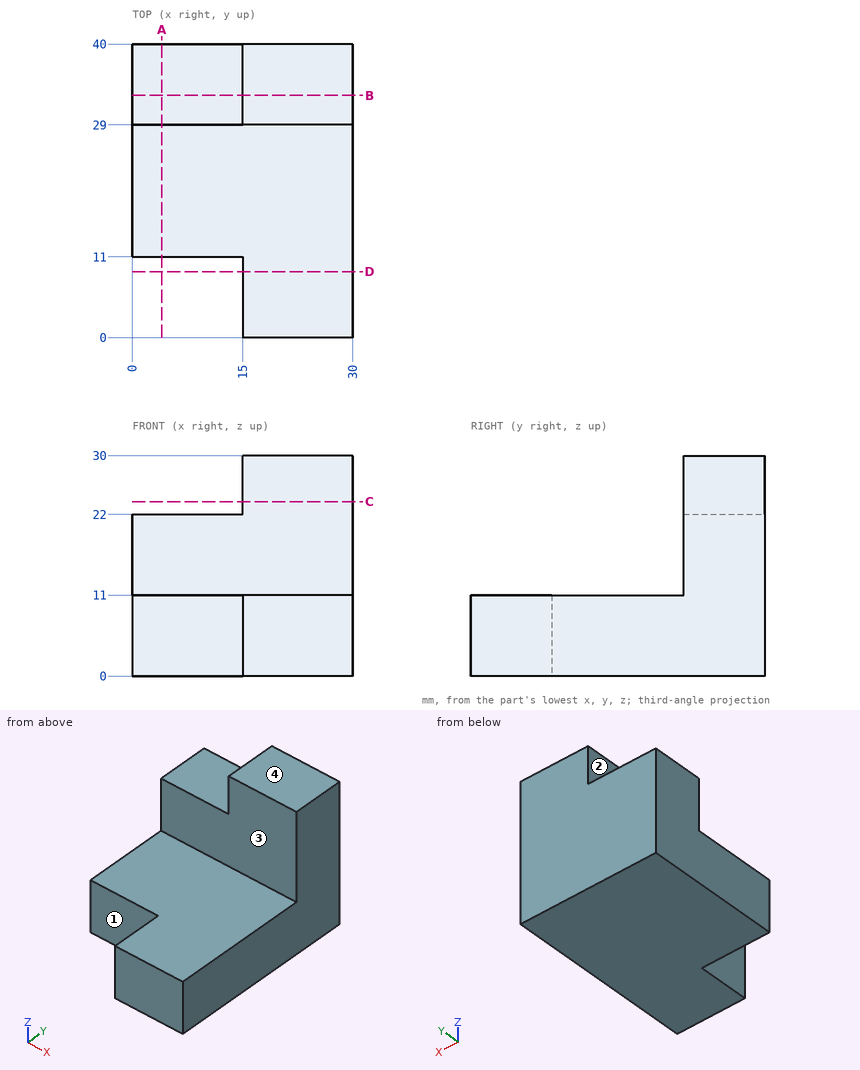
The drawing under review shows one solid part. Ordinate dimensions are in mm from its lowest x, y, z. A direction names the side the tool comes from. Round coordinates to 2 decimals unless told otherwise and drop trailing zeros. Loops run counter-clockwise (first coordinate to the right, second up) from the corner with the lowest first, then second, coordinate; pieces in that order, holes last. Notation, with made-up numbers: (50.5, 33) - (109.5, 33) arc R30 ccw to (109.5, 66) - close; hole circle Ø4 at (52, -27.75). An arc over 180 degrees is marked (long way). Put each result on its own line as item: value. Start each with the question number.
1. Consider section A-A on x = 4. State the section outline as (y, z) points.
2. For probe 1 along Z at (x, y) = (15, 18); probe 2 along Y at (x, z) = (15, 19); probe 3 along Z at (x, y) = (8, 30.5), list the stretches that pass through material, from the lowest coordinate up. Write a range as [from, to].
3. Consider section B-B on y = 33. State the section outline as (x, z) points, plus the area to 3 significant figures.
4. Consider section C-C on z = 23.75. State the section outline as (x, y) points, plus the area to 3 significant figures.
5. For the marked faces 1, 2, 3 and 4, list the 3-axis set-ups (+Z, -Z, +X, -X, +Y, -Y) from which the entire face can be reached by the end or side of a thin tool; tool diameter is ignored.
6. Consider section D-D on y = 9. State the section outline as (x, z) points, plus the area to 3 significant figures.
7. Insertion check: P1, Ø12, axis at x = 6, z = 7.5, coming from the -Y side; P2, Ø12, axis at x = 8, y = 34.5, coming from the +Z side; P3, Ø2, axis at x = 4.5, y = 16.5, coming from the +Z side. Each pin has a flat end and moves straight along its axis. Give the tip position at first contact, or say it passes through.
Result sheet:
1. outline: (11, 0) - (40, 0) - (40, 22) - (29, 22) - (29, 11) - (11, 11) - close
2. probe 1: [0, 11]
2. probe 2: [29, 40]
2. probe 3: [0, 22]
3. outline: (0, 0) - (30, 0) - (30, 30) - (15, 30) - (15, 22) - (0, 22) - close
3. area: 780 mm^2
4. outline: (15, 29) - (30, 29) - (30, 40) - (15, 40) - close
4. area: 165 mm^2
5. face 1: +Z, -Z, -X, -Y
5. face 2: +Z, -X, +Y, -Y
5. face 3: +Z, +X, -X, -Y
5. face 4: +Z, +X, -X, +Y, -Y
6. outline: (15, 0) - (30, 0) - (30, 11) - (15, 11) - close
6. area: 165 mm^2
7. P1: y = 11
7. P2: z = 22
7. P3: z = 11
